Build history of the part. All positions in model axes, mm. Face numbers are marked on the shaded views. Give positions to 0.01 mm unless a question says otherwise; leave off trailing zeros. Order: outer loops, then holes, each group sorted by start corner. A loop starts at its lowest first (then second) coordinate and runs counter-clockwise, first axis right, second up. Notation, with made-up numbers: (32, 63.25) -> (45, 63.25) arc R14 ccw to (45, 83.25) -> close; hole circle Ø8 at (-5, -16.5). An arc over 180 degrees is marked (long way). One line per item, written item: value. Start each with the question number.
(1) Saw through at C-C on z = 33.5. Give the cut face in (x, y), plus the area to 3 significant figures.
(2) Probe line 1 (Z direction, x = 103.3, y = -50); line 2 (Y direction, x = 96, z = 77); line 3 (Z direction, x = 42.45, y = -2.6). List the from-to ranges inside material, lowest first.
(3) Saw through at D-D on y = -64. Give the cut face in (x, z).
(4) Saw through at A-A on x = 96. Give the cut face in (y, z).
(5) Pin check, flat tips, straight feed: pin 1 (4 mm diameter, centred on x = 63.55, z = 28.95, fed in from +Y); pin 2 (5 mm diameter, centred on y = -124, z = 67, fed in from -X); pin 3 (5.5 mm diameter, centred on y = -50, z = 67, fed in from +X); pin 4 (2 mm diameter, centred on x = 60.5, z = 43, fed in from -Y). Stop position of each tip, or through.
(6) Saw through at B-B on y = -164. Give the cut face in (x, z).
(7) Two-plate mould, pull along Z, no slides. Class the marked faces 1, 2, 3 and 4: +Z half, -Z half, draft (parallel to the pull), parting line (faces both ways), or undercut.
```python
from build123d import *

# Parameters (mm, degrees)
F0_W            = 106
F0_H            = 75
F1_DEPTH        = 174
F2_W            = 106
F2_H            = 174
F3_DEPTH        = 4
F4_W            = 98
F4_H            = 166
F5_DEPTH        = 71
F7_D            = 4.3
F7_DEPTH        = 30
F7_CSINK_D      = 9
F7_CSINK_ANGLE  = 90
F10_D           = 4.3
F10_DEPTH       = 30
F12_D           = 4.3
F12_DEPTH       = 30
F13_D           = 4.3
F13_DEPTH       = 30
F13_CSINK_D     = 9
F13_CSINK_ANGLE = 90
F15_D           = 4.1
F15_DEPTH       = 30
F16_D           = 19
F16_DEPTH       = 40
F18_D           = 18
F18_DEPTH       = 40
F19_R           = 2


with BuildPart() as f1:
    # F0 (on Front) → F1 (new body)
    with BuildSketch(Plane.XZ):
        with Locations((53, 37.5)):
            Rectangle(F0_W, F0_H)
    extrude(amount=F1_DEPTH)

    # F2 (on face) → F3 (join)
    with BuildSketch(Plane.XY.offset(75)):
        with Locations((53, -87)):
            Rectangle(F2_W, F2_H)
        with BuildLine():
            Line((87.5, -149.5), (18.5, -149.5))
            ThreePointArc((18.5, -149.5), (14.964466, -148.035534), (13.5, -144.5))
            Line((13.5, -144.5), (13.5, -29.5))
            ThreePointArc((13.5, -29.5), (14.964466, -25.964466), (18.5, -24.5))
            Line((18.5, -24.5), (87.5, -24.5))
            ThreePointArc((87.5, -24.5), (91.035534, -25.964466), (92.5, -29.5))
            Line((92.5, -29.5), (92.5, -144.5))
            ThreePointArc((92.5, -144.5), (91.035534, -148.035534), (87.5, -149.5))
        make_face(mode=Mode.SUBTRACT)
    extrude(amount=F3_DEPTH)

    # F4 (on face) → F5 (cut)
    with BuildSketch(Plane.XY.offset(75)):
        with Locations((53, -87)):
            Rectangle(F4_W, F4_H)
    extrude(amount=-F5_DEPTH, mode=Mode.SUBTRACT)

    # F7
    with Locations(Plane.YZ.offset(106)):
        with Locations((-124, 67), (-124, 42), (-50, 67), (-50, 42)):
            CounterSinkHole(F7_D / 2, F7_CSINK_D / 2, depth=F7_DEPTH, counter_sink_angle=F7_CSINK_ANGLE)

    # F10
    with Locations(Plane.XZ.offset(174)):
        with Locations((42.45, 50.05), (42.45, 28.95), (63.55, 50.05), (63.55, 28.95)):
            Hole(F10_D / 2, depth=F10_DEPTH)

    # F12
    with Locations(Plane(origin=(0, 0, 0), x_dir=(-1, 0, 0), z_dir=(0, 1, 0))):
        with Locations((-63.55, 50.05), (-63.55, 28.95), (-42.45, 50.05), (-42.45, 28.95)):
            Hole(F12_D / 2, depth=F12_DEPTH)

    # F13
    with Locations(Plane(origin=(0, 0, 0), x_dir=(0, -1, 0), z_dir=(-1, 0, 0))):
        with Locations((50, 67), (50, 42), (124, 67), (124, 42)):
            CounterSinkHole(F13_D / 2, F13_CSINK_D / 2, depth=F13_DEPTH, counter_sink_angle=F13_CSINK_ANGLE)

    # F15
    with Locations(Plane.XY.offset(79)):
        with Locations((10, -10), (96, -10), (10, -164), (96, -164)):
            Hole(F15_D / 2, depth=F15_DEPTH)

    # F16
    with Locations(Plane.XZ.offset(174)):
        with Locations((53, 39.5)):
            Hole(F16_D / 2, depth=F16_DEPTH)

    # F18
    with Locations(Plane(origin=(0, 0, 0), x_dir=(-1, 0, 0), z_dir=(0, 1, 0))):
        with Locations((-53, 39.5)):
            Hole(F18_D / 2, depth=F18_DEPTH)

    # F19
    f19_edges = [f1.edges().sort_by_distance(p)[0] for p in [
        (0, 0, 39.5),
        (106, 0, 39.5),
        (106, -174, 39.5),
        (0, -174, 39.5),
        (53, -174, 0),
        (0, -87, 0),
        (53, 0, 0),
        (106, -87, 0),
    ]]
    fillet(f19_edges, radius=F19_R)


solid = f1.part
```
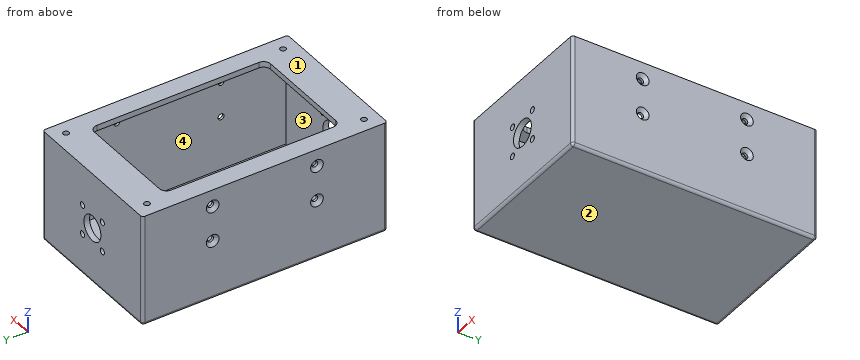
Results below:
1. outline: (0, -172) arc R2 ccw to (2, -174) -> (45.63, -174) -> (45.63, -170) -> (4, -170) -> (4, -4) -> (46.29, -4) -> (46.29, 0) -> (2, 0) arc R2 ccw to (0, -2) -> close; (59.71, -4) -> (102, -4) -> (102, -170) -> (60.37, -170) -> (60.37, -174) -> (104, -174) arc R2 ccw to (106, -172) -> (106, -2) arc R2 ccw to (104, 0) -> (59.71, 0) -> close
1. area: 2,060 mm²
2. line 1: z = 0 to 39.85, 44.15 to 64.85, 69.15 to 79
2. line 2: y = -174 to -166.05, -161.95 to -12.05, -7.95 to 0
2. line 3: z = 0 to 26.8, 31.1 to 47.9, 52.2 to 79
3. outline: (0, 2) arc R2 ccw to (2, 0) -> (104, 0) arc R2 ccw to (106, 2) -> (106, 79) -> (92.5, 79) -> (92.5, 75) -> (102, 75) -> (102, 4) -> (4, 4) -> (4, 75) -> (13.5, 75) -> (13.5, 79) -> (0, 79) -> close
4. outline: (-174, 2) arc R2 ccw to (-172, 0) -> (-2, 0) arc R2 ccw to (0, 2) -> (0, 79) -> (-7.95, 79) -> (-7.95, 75) -> (-4, 75) -> (-4, 4) -> (-170, 4) -> (-170, 75) -> (-166.05, 75) -> (-166.05, 79) -> (-174, 79) -> close; (-161.95, 75) -> (-12.05, 75) -> (-12.05, 79) -> (-161.95, 79) -> close
5. pin 1: passes through
5. pin 2: stops at x = 2
5. pin 3: stops at x = 104.25
5. pin 4: stops at y = -4
6. outline: (0, 2) arc R2 ccw to (2, 0) -> (104, 0) arc R2 ccw to (106, 2) -> (106, 79) -> (98.05, 79) -> (98.05, 75) -> (102, 75) -> (102, 4) -> (4, 4) -> (4, 75) -> (7.95, 75) -> (7.95, 79) -> (0, 79) -> close; (12.05, 75) -> (93.95, 75) -> (93.95, 79) -> (12.05, 79) -> close
7. face 1: +Z half
7. face 2: -Z half
7. face 3: undercut
7. face 4: undercut
